Could you check a few things on this drawing? It's one solid part, dimensions in mm from its lowest x, y, z. Coordinates: 2 decimals unless noted, no trailing zeros. Loops run counter-clockwise (first coordinate to the right, second up) from the corner with the lowest first, then second, coordinate; pieces in that order, holes last. Notation, with made-up numbers: (-36, 13.25) -> (-26, 13.25) arc R28 ccw to (-26, 35.25) -> close; hole circle Ø2 at (53, -24.75). An arc over 180 degrees is marked (long way). One line per question, with ' | ' between items.
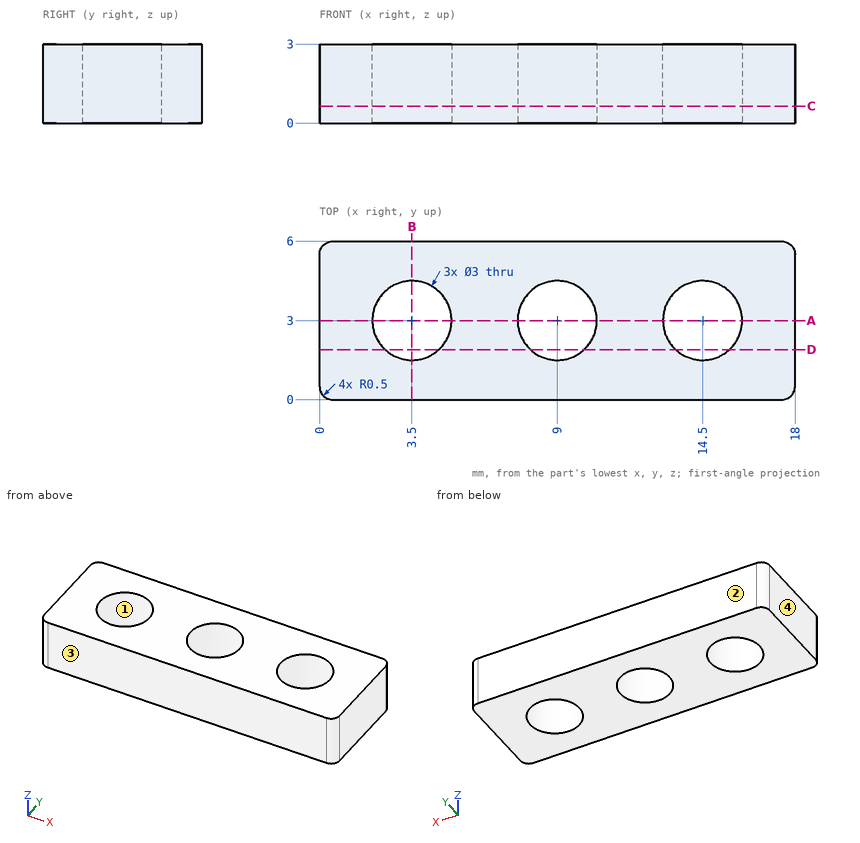
1) We'd pull the mould along Y, two halves only. Please class the marked faces 1, 2, 3 and 4: pulls with the +Y half, pulls with the -Y half, needs draft (parallel to the pull), parting line crosses it, or undercut.
Data:
face 1: undercut | face 2: pulls with the +Y half | face 3: pulls with the -Y half | face 4: needs draft
2) I need wall thicknesses on line 1 along X through (y, z) = (2.9, 0.8); line 2 along X through (y, z) = (3.55, 1.7); line 3 along Y through (x, z) = (3.5, 1.1). Which ranges of each line are inside material? Lowest first, please. Write a range as from..to.
Data:
line 1: 0..2, 5..7.5, 10.5..13, 16..18 | line 2: 0..2.1, 4.9..7.6, 10.4..13.1, 15.9..18 | line 3: 0..1.5, 4.5..6
3) If we section it at B-B on x = 3.5: Please give me the cut outline in (y, z).
Data:
outline: (0, 0) -> (1.5, 0) -> (1.5, 3) -> (0, 3) -> close; (4.5, 0) -> (6, 0) -> (6, 3) -> (4.5, 3) -> close
4) If we section it at D-D on y = 1.9: Please give me the cut outline in (x, z).
Data:
outline: (0, 0) -> (2.48, 0) -> (2.48, 3) -> (0, 3) -> close; (4.52, 0) -> (7.98, 0) -> (7.98, 3) -> (4.52, 3) -> close; (10.02, 0) -> (13.48, 0) -> (13.48, 3) -> (10.02, 3) -> close; (15.52, 0) -> (18, 0) -> (18, 3) -> (15.52, 3) -> close
5) I'm going to push a flat-ended pin straight in: pin 1 Ø1 at (y, z) = (3.5, 1) entering from -X. Where does the tip first touch, or does it pass through?
Data:
pin 1: x = 0
6) If we section it at A-A on y = 3: Please give me the cut outline in (x, z).
Data:
outline: (0, 0) -> (2, 0) -> (2, 3) -> (0, 3) -> close; (5, 0) -> (7.5, 0) -> (7.5, 3) -> (5, 3) -> close; (10.5, 0) -> (13, 0) -> (13, 3) -> (10.5, 3) -> close; (16, 0) -> (18, 0) -> (18, 3) -> (16, 3) -> close
7) If we section it at C-C on z = 0.65: Please give me the cut outline in (x, y).
Data:
outline: (0, 0.5) arc R0.5 ccw to (0.5, 0) -> (17.5, 0) arc R0.5 ccw to (18, 0.5) -> (18, 5.5) arc R0.5 ccw to (17.5, 6) -> (0.5, 6) arc R0.5 ccw to (0, 5.5) -> close; hole circle Ø3 at (3.5, 3); hole circle Ø3 at (9, 3); hole circle Ø3 at (14.5, 3)
